from build123d import *

# Parameters (mm, degrees)
F3_DEPTH = 25.4
F4_COUNT = 4
F5_R     = 6.35
F6_DEPTH = 508


with BuildPart() as f1:
    # F0 (on Front) → F1 (revolve)
    with BuildSketch(Plane.XZ):
        Polygon((-76.2, 152.4), (0, 152.4), (0, 177.8), (-127, 177.8), (-127, 254), (-152.4, 254), (-152.4, 152.4), align=None)
        Polygon((-152.4, 0), (0, 0), (0, 152.4), (-76.2, 152.4), align=None)
    revolve(axis=Axis((0, 0, 76.2), (0, 0, -1)))

    # F2 (on Front) → F3 (join, symmetric)
    with BuildSketch(Plane.XZ):
        Polygon((177.8, 0), (25.4, 0), (67.2867714516, -50.8), (153.8449790805, -50.8), (237.6185219837, -152.4), (303.4603143548, -152.4), align=None)
    extrude(amount=F3_DEPTH, both=True)

    # F4: F1 ×4 about axis
    f4_axis = Axis((0, 0, 152.4), (0, 0, -1))


with BuildPart() as f1_1:
    add(f1.part)
    for i in range(1, F4_COUNT):
        add(f1.part.rotate(f4_axis, i * 360 / F4_COUNT))

    # F5 (on Front) → F6 (cut)
    with BuildSketch(Plane.XZ):
        with Locations((0, 203.2)):
            Circle(F5_R)
    extrude(amount=-F6_DEPTH, mode=Mode.SUBTRACT)


solid = f1_1.part
Work out the finished part from the listing and answer in its coordinate system (mm). A direction names the side the tool comes from. Give positions to 0.01 mm unless a question says otherwise; leave off trailing zeros. Order: outer loops, then holes, each group sorted by start corner. A loop starts at its lowest first (then second) coordinate and runs counter-clockwise, first axis right, second up. Notation, with made-up numbers: M 33,-2.75 L 55,-2.75 A13 ccw 55,2.25 Z; hole C 29.25,37 d6. An arc over 180 degrees is marked long. Return JSON: item names as keys, results as strings.
Q1. Find section A-A, the plane z = -73. Write down the section's boundary in (x, y).
Answer below:
{"outline": "M -237.99,-25.4 L -172.15,-25.4 L -172.15,25.4 L -237.99,25.4 Z; M -25.4,-237.99 L 25.4,-237.99 L 25.4,-172.15 L -25.4,-172.15 Z; M -25.4,172.15 L 25.4,172.15 L 25.4,237.99 L -25.4,237.99 Z; M 172.15,-25.4 L 237.99,-25.4 L 237.99,25.4 L 172.15,25.4 Z"}
Q2. Find section D-D, the plane x = -257.5. Write down the section's boundary in (y, z), and give its area (3 significant figures).
Answer below:
{"outline": "M -25.4,-152.4 L 25.4,-152.4 L 25.4,-96.66 L -25.4,-96.66 Z", "area": "2,830 mm^2"}
Q3. Find the intervals of material crossed by line 1 along Y through (x, z) = (0, 210); line 2 along Z through (x, y) = (0, 133.75); line 3 along Y through (x, z) = (0, 201), in increasing order. Write a range as [from, to].
Answer below:
{"line 1": "y = [-152.4, -127], [127, 152.4]", "line 2": "z = [-50.8, 37.3], [152.4, 196.85], [209.55, 254]", "line 3": "y = [-152.4, -127]"}
Q4. Which of the six approach directions +Z, -Z, +X, -X, +Y, -Y give full straight-line access (tool end or side, diameter ignored) to faces 4 (the face through (75, -73, 0)), 5 (the face through (0.356, 195.145, -100.889)), 6 (the face through (-32, 70, 152.4))?
Answer below:
{"face 4": "-Z, +X, -Y", "face 5": "-Z, +X, -X", "face 6": "none"}
Q5. The mould has two halves that part along X. Classify faces 1 (the face through (-241.51, 0.36, -77.27)), 2 (the face through (46.05, -0.356, -25.044)), 3 (the face through (-174, -25.4, -65)): pulls with the +X half, pulls with the -X half, needs draft (parallel to the pull), parting line crosses it, or undercut.
Answer below:
{"face 1": "pulls with the -X half", "face 2": "undercut", "face 3": "needs draft"}
Q6. Each of these flat-tipped pins is pushed along its axis until it touches: pin 1 (2 mm diameter, centred on y = -31.5, z = 178, fed in from +X); pin 2 (5 mm diameter, centred on y = 172, z = -7, fed in from +X); pin 3 (6 mm diameter, centred on y = 102.5, z = 57, fed in from -X). Where does it stop, or does it pass through?
Answer below:
{"pin 1": "stops at x = 149.32", "pin 2": "stops at x = 25.4", "pin 3": "stops at x = -74.55"}
Q7. Find section B-B, the plane y = 0. Write down the section's boundary in (x, z).
Answer below:
{"outline": "M -303.46,-152.4 L -237.62,-152.4 L -153.84,-50.8 L -67.29,-50.8 L -25.4,0 L 25.4,0 L 67.29,-50.8 L 153.84,-50.8 L 237.62,-152.4 L 303.46,-152.4 L 177.8,0 L 152.4,0 L 76.2,152.4 L 152.4,152.4 L 152.4,254 L 127,254 L 127,177.8 L -127,177.8 L -127,254 L -152.4,254 L -152.4,152.4 L -76.2,152.4 L -152.4,0 L -177.8,0 Z"}
Q8. Find section C-C, the plane z = 18. Write down the section's boundary in (x, y), and give its area (3 significant figures).
Answer below:
{"outline": "C 0,0 d286.8", "area": "64,600 mm^2"}
